Autodesk Inventor part; units mm, degrees
ref_plane "YZ Plane" through (0, 0, 0) normal (1, 0, 0) x (0, 1, 0)
ref_plane "XZ Plane" through (0, 0, 0) normal (0, 1, 0) x (-1, 0, 0)
ref_plane "XY Plane" through (0, 0, 0) normal (0, 0, 1) x (1, 0, 0)
sketch "Sketch1" plane through (0, 0, 0) normal (0, 1, 0) x (-1, 0, 0)
  line L0 (0, 0) -> (0, -30)
  line L1 (0, 0) -> (0.75, 0) construction
  arc A0 (1.4548, 0.2565) -> (0, 0) centre (0.75, 0) ccw
  line L2 (1.4548, 0.2565) -> (6.5322, -13.6936)
  line L3 (0, -30) -> (0.75, -30) construction
  circle A1 centre (0.75, -30) radius 0.75
  line L4 (1.0065, -30.7048) -> (6.5322, -28.6936)
  line L5 (6.5322, -13.6936) -> (6.5322, -28.6936) construction
  line L6 (6.5322, -13.6936) -> (35.2454, -42.4068)
  line L7 (6.5322, -13.6936) -> (66.5322, -13.6936) construction
  line L8 (6.5322, -28.6936) -> (27.7454, -49.9068)
  line L9 (6.5322, -28.6936) -> (36.5322, -28.6936) construction
  line L10 (27.7454, -49.9068) -> (27.7454, -64.9068)
  line L11 (27.7454, -64.9068) -> (6.5322, -86.12)
  line L12 (27.7454, -64.9068) -> (57.7454, -64.9068) construction
  line L13 (35.2454, -42.4068) -> (27.7454, -49.9068) construction
  arc A2 (36.7987, -46.1568) -> (35.2454, -42.4068) centre (31.4954, -46.1568) ccw
  line L14 (36.7987, -46.1568) -> (36.7987, -68.6568)
  line L15 (27.7454, -64.9068) -> (27.7454, -79.9068) construction
  line L16 (27.7454, -79.9068) -> (16.5322, -91.12)
  line L17 (27.7454, -79.9068) -> (35.2454, -72.4068)
  line L18 (27.7454, -64.9068) -> (35.2454, -72.4068) construction
  arc A3 (35.2454, -72.4068) -> (36.7987, -68.6568) centre (31.4954, -68.6568) ccw
  line L19 (6.5322, -86.12) -> (16.5322, -86.12) construction
  line L20 (16.5322, -86.12) -> (16.5322, -91.12) construction
  line L21 (16.5322, -116.12) -> (6.5322, -116.12)
  line L22 (6.5322, -116.12) -> (6.5322, -86.12)
  line L23 (16.5322, -91.12) -> (16.5322, -116.12)
  circle A4 centre (11.5322, -93.62) radius 2
  circle A5 centre (11.5322, -108.62) radius 2
  line L24 (0, -3.6658) -> (-2.5, -3.6658)
  line L25 (-2.5, -3.6658) -> (-2.5, -6.1658)
  line L26 (-2.5, -6.1658) -> (0, -6.1658)
  line L27 (0, -6.1658) -> (0, -3.6658)
  line L28 (-2.5, -3.6658) -> (0, -2.5)
  line L29 (-2.5, -6.1658) -> (0, -7.3315)
  line L30 (0, -10.9973) -> (-2.5, -10.9973)
  line L31 (-2.5, -10.9973) -> (-2.5, -13.4973)
  line L32 (-2.5, -13.4973) -> (0, -13.4973)
  line L33 (-2.5, -10.9973) -> (0, -9.8315)
  line L34 (-2.5, -13.4973) -> (0, -14.6631)
  line L35 (-2.5, -18.3288) -> (-2.5, -20.8288)
  line L36 (-2.5, -20.8288) -> (0, -21.9946)
  line L37 (-2.5, -20.8288) -> (0, -20.8288)
  line L38 (0, -18.3288) -> (-2.5, -18.3288)
  line L39 (-2.5, -18.3288) -> (0, -17.1631)
  line L40 (-2.5, -25.6604) -> (0, -24.4946)
  line L41 (0, -25.6604) -> (-2.5, -25.6604)
  line L42 (-2.5, -25.6604) -> (-2.5, -28.1604)
  line L43 (-2.5, -28.1604) -> (0, -28.1604)
  line L44 (-2.5, -28.1604) -> (0, -29.3262)
  circle A6 centre (6.5322, -21.1936) radius 2
  circle A7 centre (31.4954, -46.1568) radius 2
  circle A8 centre (31.4954, -68.6568) radius 2
  dimension "d2" = 30
  dimension "d17" = 0.75
  dimension "d18" = 20
  dimension "d19" = 0.75
  dimension "d20" = 70
  dimension "d21" = 15
  dimension "d28" = 45
  dimension "d29" = 30
  dimension "d30" = 45
  dimension "d31" = 15
  dimension "d34" = 135
  dimension "d35" = 15
  dimension "d36" = 135
  dimension "d38" = 10
  dimension "d39" = 30
  dimension "d40" = 30
  dimension "d41" = 7.5
  dimension "d42" = 5
  dimension "d43" = 7.5
  dimension "d44" = 5
  dimension "d45" = 4
  dimension "d46" = 4
  dimension "d47" = 2.5
  dimension "d48" = 2.5
  dimension "d49" = 25
  dimension "d50" = 25
  dimension "d51" = 2.5
  dimension "d52" = 2.5
  dimension "d53" = 2.5
  dimension "d54" = 25
  dimension "d55" = 25
  dimension "d56" = 2.5
  dimension "d57" = 2.5
  dimension "d58" = 2.5
  dimension "d59" = 25
  dimension "d60" = 25
  dimension "d61" = 2.5
  dimension "d62" = 2.5
  dimension "d63" = 2.5
  dimension "d64" = 25
  dimension "d65" = 25
  dimension "d66" = 2.5
  dimension "d69" = 4
  dimension "d70" = 4
  dimension "d71" = 4
extrude "Extrusion2" add sketch "Sketch1" along normal blind 2
properties part number "claw_gripper"
Can you work these out from the model? Positions are in its coordinate system, mm. A direction names the side the tool comes from. Round coordinates to 2 decimals unless told otherwise and drop trailing zeros. Order: outer loops, then holes, each group sorted by start corner. A loop starts at its lowest first (then second) coordinate and runs counter-clockwise, first axis right, second up. Notation, with made-up numbers: M 28,43 L 74,43 A22 cw 74,68 Z; hole C 62,83 d6. An arc over 180 degrees is marked long. Use a Markdown table: item, result.
1) Imagine slicing it at C-C (z = -75.5). List the corners of the cut face in (x, y) for me, then the cut area to 3 significant figures.
Geometry says:
| item | result |
|---|---|
| outline | M -32.15,0 L -17.15,0 L -17.15,2 L -32.15,2 Z |
| area | 30.0 mm² |
2) If we mould it in two halves opening along Z, with no side actions, what happens to faces 3 (the face through (0, 1, -1)), 4 (the face through (-12, 1, -116.12)), 5 (the face through (-17.29, 0.99, -75.36))? For each: +Z half, -Z half, draft (parallel to the pull), parting line (faces both ways), or undercut.
Geometry says:
| item | result |
|---|---|
| face 3 | draft |
| face 4 | -Z half |
| face 5 | undercut |
3) If I drill on line 1 along Z through (x, y) = (-11, 1.7); line 2 along X through (y, z) = (0.85, -105); line 3 along Z through (x, y) = (-10, 0.45), over which ranges is the centre line in solid material (lowest first)?
Geometry says:
| item | result |
|---|---|
| line 1 | z = -116.12 to -110.55, -106.69 to -95.55, -91.69 to -81.65, -33.16 to -18.16 |
| line 2 | x = -16.53 to -6.53 |
| line 3 | z = -116.12 to -109.91, -107.33 to -94.91, -92.33 to -82.65, -32.16 to -17.16 |
4) I'm going to push flat-ended pins straight in: P1, Ø0.6, axis at y = 0.5, z = -8, coming from the +X side; P2, Ø0.6, axis at y = 1, z = -56.5, coming from the +X side; P3, Ø0.6, axis at y = 1, z = -98, coming from the +X side. Where does each tip first touch, or does it pass through?
Geometry says:
| item | result |
|---|---|
| P1 | stops at x = 0 |
| P2 | stops at x = -27.75 |
| P3 | stops at x = -6.53 |
5) On a 3-axis mill with a long thin cutter (end or side, diameter ignored), from which of +Z, -Z, +X, -X, +Y, -Y can I reach the whole of each face in a straight line? I mean faces 1 (the face through (1.27, 0.99, -6.74)), 2 (the face through (1.267, 0.986, -3.091)). Say none if no direction works.
Geometry says:
| item | result |
|---|---|
| face 1 | +X, +Y, -Y |
| face 2 | +Z, +X, +Y, -Y |
6) Imagine slicing it at B-B (y = 1.5). Give the number of separate pieces and of enclosed holes in the cut face, then the cut area to 3 significant figures.
Geometry says:
| item | result |
|---|---|
| separate pieces | 1 |
| enclosed holes | 5 |
| area | 1,300 mm² |
7) Imagine slicing it at A-A (z = -93.62). List the corners of the cut face in (x, y) for me.
Geometry says:
| item | result |
|---|---|
| outline | M -16.53,0 L -13.53,0 L -13.53,2 L -16.53,2 Z; M -9.53,0 L -6.53,0 L -6.53,2 L -9.53,2 Z |
